Work out the finished part from the listing and answer in its coordinate system (mm). Coordinates: 2 decimals unless noted, no trailing zeros. Order: outer loops, then holes, each group sorted by start corner. A loop starts at its lowest first (then second) coordinate and runs counter-clockwise, first axis right, second up. Notation, with made-up numbers: M -5,-5 L 46,-5 A17 ccw 46,28 Z; hole C -11.75,80.25 d6. An arc over 180 degrees is marked long. Use a Markdown table: item, result.
Autodesk Inventor part; units mm, degrees
ref_plane "Work Plane2" through (0, -7.5, 0) normal (-1, 0, 0) x (0, 0, 1)
ref_plane "YZ Plane" through (0, 0, 0) normal (1, 0, 0) x (0, 1, 0)
ref_plane "XZ Plane" through (0, 0, 0) normal (0, 1, 0) x (-1, 0, 0)
sketch "Sketch1" plane through (0, 0, 0) normal (0, 0, 1) x (1, 0, 0)
  line L0 (55, -22.5) -> (-55, -22.5)
  line L1 (-55, -22.5) -> (-55, 22.5)
  line L2 (-55, 22.5) -> (55, 22.5)
  line L3 (55, 22.5) -> (55, -22.5)
  line L4 (55, -22.5) -> (-55, 22.5) construction
  line L5 (-55, -22.5) -> (55, 22.5) construction
  point P0 (0, 0)
  dimension "d0" = 110
  dimension "d1" = 45
extrude "Extrusion1" add sketch "Sketch1" along normal blind 4
sketch "Sketch2" plane through (0, 0, 4) normal (0, 0, 1) x (1, 0, 0)
  line L0 (-55, 22.5) -> (-55, -22.5)
  line L1 (-55, 17.5) -> (-51, 17.5)
  line L2 (-51, 17.5) -> (-51, 7.5)
  line L3 (-51, 7.5) -> (-55, 7.5)
  line L4 (-55, 7.5) -> (-55, 17.5)
  line L5 (-55, -7.5) -> (-51, -7.5)
  line L6 (-51, -7.5) -> (-51, -17.5)
  line L7 (-51, -17.5) -> (-55, -17.5)
  line L8 (-55, -17.5) -> (-55, -7.5)
  line L9 (55, 22.5) -> (-55, 22.5)
  line L10 (-55, -22.5) -> (55, -22.5)
  point P0 (0, 0)
  dimension "d4" = 4
  dimension "d5" = 10
  dimension "d6" = 4
  dimension "d7" = 10
  dimension "d8" = 5
  dimension "d9" = 5
extrude "Extrusion2" cut sketch "Sketch2" against normal blind 4
ref_plane "Work Plane2" through (0, -7.5, 0) normal (-1, 0, 0) x (0, 0, 1)
mirror "Mirror1" about plane through (0, -7.5, 0) normal (-1, 0, 0) of "Extrusion2"
properties part number "FUENTE 1"
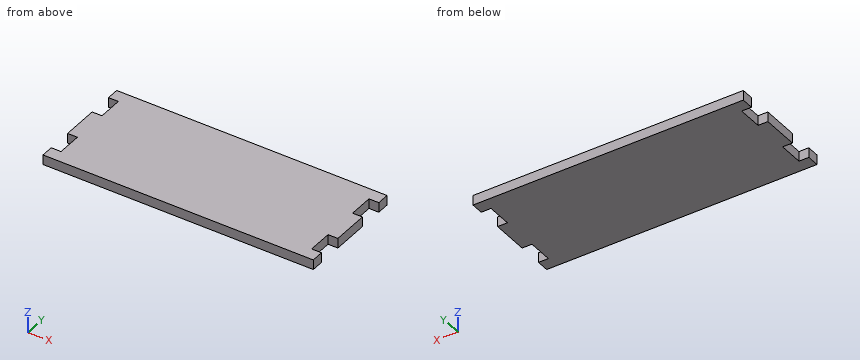
1. Find the intervals of material crossed by probe 1 along X at (y, z) = (-8, 0.65), in increasing order.
Answers below:
| item | result |
|---|---|
| probe 1 | -51 to 51 |
2. Section B-B on y = 15 is taken. Determine the outline of the cut face in (x, z), then the cut area to 3 significant figures.
Answers below:
| item | result |
|---|---|
| outline | M -51,0 L 51,0 L 51,4 L -51,4 Z |
| area | 408 mm² |
3. A flat-ended cylindrical pin translates along its axis: P1, Ø2, axis at y = -13.5, z = 3, coming from the +X side. Find the tip coordinate at first contact, or state that the pin passes through.
Answers below:
| item | result |
|---|---|
| P1 | x = 51 |
4. Section A-A on z = 0.9 is taken. Determine the outline of the cut face in (x, y).
Answers below:
| item | result |
|---|---|
| outline | M -55,-22.5 L 55,-22.5 L 55,-17.5 L 51,-17.5 L 51,-7.5 L 55,-7.5 L 55,7.5 L 51,7.5 L 51,17.5 L 55,17.5 L 55,22.5 L -55,22.5 L -55,17.5 L -51,17.5 L -51,7.5 L -55,7.5 L -55,-7.5 L -51,-7.5 L -51,-17.5 L -55,-17.5 Z |
